Answer from the drawing. Dimensions are ordinates in mm from the lowest x, y and z of the part. Coordinates: 2 decimals unless noted, no trailing zeros. Order: outer loops, then holes, each group sorted by start corner. A loop starts at its lowest first (then second) coordinate and runs counter-clockwise, first axis right, second up. Notation, with made-up numbers: (-15.75, 35) -> (-0.75, 35) arc R14 cw to (-0.75, 50) -> close; hole circle Ø4 at (-32, -23). An arc over 180 degrees is marked (long way). Use CSV: the item, a comma, the result in double quotes.
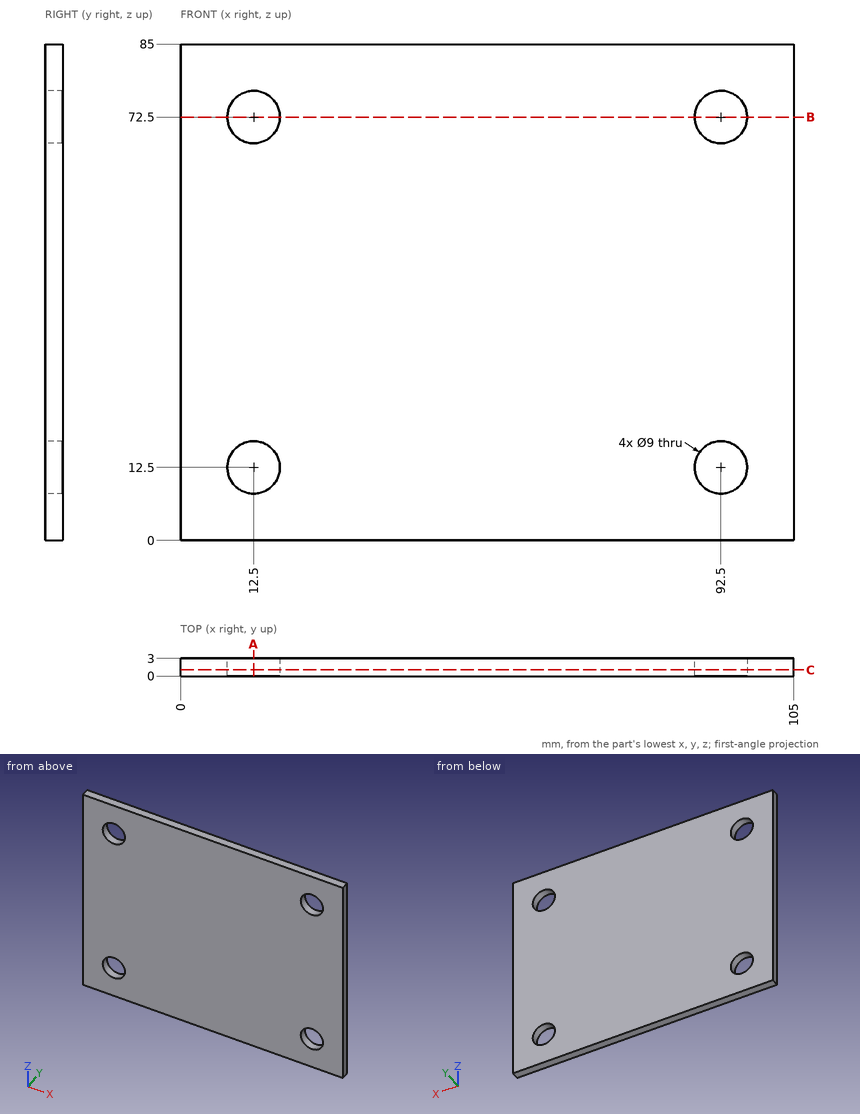
Item 1: Find section C-C, the plane y = 1.05. Give the vertices of the cut face in (x, z).
Return value:
outline,"(0, 0) -> (105, 0) -> (105, 85) -> (0, 85) -> close; hole circle Ø9 at (12.5, 12.5); hole circle Ø9 at (12.5, 72.5); hole circle Ø9 at (92.5, 12.5); hole circle Ø9 at (92.5, 72.5)"
Item 2: This flat-tipped pin is pushed along its axis until it touches: P1, Ø5.5, axis at x = 12.5, z = 12.5, coming from the +Y side. Where does it stop, or does it pass through?
Return value:
P1,"passes through"
Item 3: Find section B-B, the plane z = 72.5. Give the vertices of the cut face in (x, y), then the cut area to 3 significant figures.
Return value:
outline,"(0, 0) -> (8, 0) -> (8, 3) -> (0, 3) -> close; (17, 0) -> (88, 0) -> (88, 3) -> (17, 3) -> close; (97, 0) -> (105, 0) -> (105, 3) -> (97, 3) -> close"
area,"261 mm^2"
Item 4: Find section A-A, the plane x = 12.5. Give the vertices of the cut face in (y, z).
Return value:
outline,"(0, 0) -> (3, 0) -> (3, 8) -> (0, 8) -> close; (0, 17) -> (3, 17) -> (3, 68) -> (0, 68) -> close; (0, 77) -> (3, 77) -> (3, 85) -> (0, 85) -> close"
Item 5: Straight lines are drawn through the part: line 1 along Z through (x, y) = (12.5, 1.45); line 2 along X through (y, z) = (0.75, 12.5); line 3 along Z through (x, y) = (89, 1.1). For each, find the intervals that lie inside material, in ascending order.
Return value:
line 1,"z = 0 to 8, 17 to 68, 77 to 85"
line 2,"x = 0 to 8, 17 to 88, 97 to 105"
line 3,"z = 0 to 9.67, 15.33 to 69.67, 75.33 to 85"
